Design review of the part built by this model. Coordinates are the model's own, in mm. Face numbers are marked on the shaded views. A direction names the side the tool comes from. Give positions to 0.01 mm unless a question says otherwise; leave off trailing zeros. Order: outer loops, then holes, each group sorted by start corner. A loop starts at its lowest first (then second) coordinate and runs counter-clockwise, first axis right, second up.
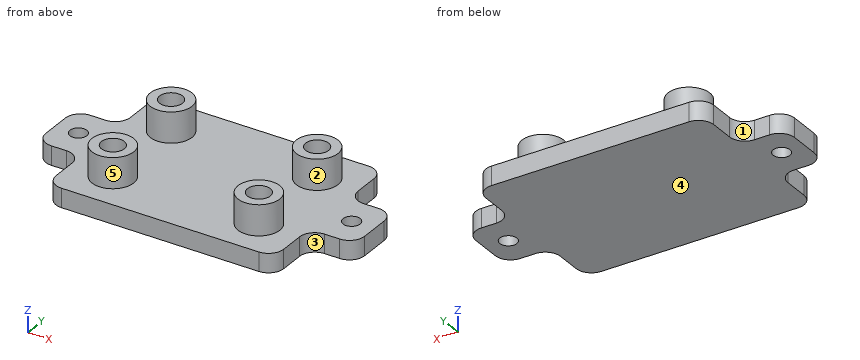
```python
from build123d import *

# Parameters (mm, degrees)
SKETCH1_W            = 60
SKETCH1_H            = 45
BOSS_EXTRUDE1_DEPTH  = 5
SKETCH3_R            = 5.5
SKETCH3_R_2          = 3.025
BOSS_EXTRUDE2_DEPTH  = 8
SKETCH4_W            = 12
SKETCH4_H            = 16
SKETCH4_R            = 2.55
BOSS_EXTRUDE3_DEPTH  = 5
FILLET1_R            = 4
M4_CLEARANCE_HOLE1_D = 4.5
MIRROR1_OUTLINE_R    = 2.25
MIRROR1_DEPTH        = 5
FILLET2_R            = 4


# Read off the part's stored shape, not the designer's step: Mirror1
with BuildPart() as part:
    # Sketch1 → Boss-Extrude1 (new body)
    with BuildSketch(Plane.XY):
        Rectangle(SKETCH1_W, SKETCH1_H)
    extrude(amount=BOSS_EXTRUDE1_DEPTH)

    # Sketch3 → Boss-Extrude2 (add)
    # profile 1 of 4: a face of its own
    with BuildSketch(Plane.XY.offset(5)):
        with Locations((-19.2405, 11.938)):
            Circle(SKETCH3_R)
        with Locations((-19.2405, 11.938)):
            Circle(SKETCH3_R_2, mode=Mode.SUBTRACT)
    # profile 2 of 4: a face of its own
    with BuildSketch(Plane.XY.offset(5)):
        with Locations((-19.2405, -11.938)):
            Circle(SKETCH3_R)
        with Locations((-19.2405, -11.938)):
            Circle(SKETCH3_R_2, mode=Mode.SUBTRACT)
    # profile 3 of 4: a face of its own
    with BuildSketch(Plane.XY.offset(5)):
        with Locations((19.2405, 11.938)):
            Circle(SKETCH3_R)
        with Locations((19.2405, 11.938)):
            Circle(SKETCH3_R_2, mode=Mode.SUBTRACT)
    # profile 4 of 4: a face of its own
    with BuildSketch(Plane.XY.offset(5)):
        with Locations((19.2405, -11.938)):
            Circle(SKETCH3_R)
        with Locations((19.2405, -11.938)):
            Circle(SKETCH3_R_2, mode=Mode.SUBTRACT)
    extrude(amount=BOSS_EXTRUDE2_DEPTH)

    # Sketch4 → Boss-Extrude3 (add)
    # profile 1 of 2: a face of its own
    with BuildSketch(Plane.XY.offset(5)):
        with Locations((-36, 0)):
            Rectangle(SKETCH4_W, SKETCH4_H)
        with Locations((-36, 0)):
            Circle(SKETCH4_R, mode=Mode.SUBTRACT)
    # profile 2 of 2: a face of its own
    with BuildSketch(Plane.XY.offset(5)):
        with Locations((-36, 0)):
            Circle(SKETCH4_R)
    extrude(amount=-BOSS_EXTRUDE3_DEPTH)

    # Fillet1
    fillet1_edges = [part.edges().sort_by_distance(p)[0] for p in [
        (-42, -8, 2.5),
        (-42, 8, 2.5),
        (-30, 8, 2.5),
        (-30, -8, 2.5),
        (-30, 22.5, 2.5),
        (-30, -22.5, 2.5),
    ]]
    fillet(fillet1_edges, radius=FILLET1_R)

    # M4 Clearance Hole1 (through all)
    with Locations(Plane.XY.offset(5)):
        with Locations((-36, 0)):
            Hole(M4_CLEARANCE_HOLE1_D / 2)

    # Mirror1 outline → Mirror1 (add)
    with BuildSketch(Plane.XY):
        with BuildLine():
            ThreePointArc((42, 4), (40.828427125, 6.828427125), (38, 8))
            Line((38, 8), (30, 8))
            Line((30, 8), (30, -8))
            Line((30, -8), (38, -8))
            ThreePointArc((38, -8), (40.828427125, -6.828427125), (42, -4))
            Line((42, -4), (42, 4))
        make_face()
        with Locations((36, 0)):
            Circle(MIRROR1_OUTLINE_R, mode=Mode.SUBTRACT)
    extrude(amount=MIRROR1_DEPTH)

    # Fillet2
    fillet2_edges = [part.edges().sort_by_distance(p)[0] for p in [
        (30, -8, 2.5),
        (30, 8, 2.5),
        (30, 22.5, 2.5),
        (30, -22.5, 2.5),
    ]]
    fillet(fillet2_edges, radius=FILLET2_R)


solid = part.part
```
1. For line 1 along Y through (x, z) = (36, 1.2); line 2 along X through (y, z) = (1, 2.25); line 3 along X through (y, z) = (-13.5, 1), list the stretches that pass through material, from the lowest coordinate up.
Recorded:
line 1: y = -8 to -2.25, 2.25 to 8
line 2: x = -42 to -38.02, -33.98 to 33.98, 38.02 to 42
line 3: x = -30 to 30
2. Take a section at C-C (z = 7.25). State how many separate pieces and enclosed holes the cut face has, then the cut area to 3 significant figures.
Recorded:
separate pieces: 4
enclosed holes: 4
area: 265 mm2
3. Take a section at D-D (y = -16). State the section outline as (x, z) points.
Recorded:
outline: (-30, 0) - (30, 0) - (30, 5) - (22.95, 5) - (22.95, 13) - (15.53, 13) - (15.53, 5) - (-15.53, 5) - (-15.53, 13) - (-22.95, 13) - (-22.95, 5) - (-30, 5) - close
4. Draft analysis for pull direction Y (two halves, no side actions). For the marked faces 3, 4 and 5, state which applies: pulls with the +Y half, pulls with the -Y half, needs draft (parallel to the pull), parting line crosses it, or undercut.
Recorded:
face 3: pulls with the -Y half
face 4: needs draft
face 5: undercut
5. Take a section at B-B (y = 0). State the section outline as (x, z) points, then the cut area to 3 significant figures.
Recorded:
outline: (-42, 0) - (-38.25, 0) - (-38.25, 5) - (-42, 5) - close; (-33.75, 0) - (33.75, 0) - (33.75, 5) - (-33.75, 5) - close; (38.25, 0) - (42, 0) - (42, 5) - (38.25, 5) - close
area: 375 mm2
6. For pin 1 (1.5 mm diameter, centred on y = -15, z = 1.5, fed in from +X); pin 2 (6.5 mm diameter, centred on x = -18, y = -11.5, fed in from +Z); pin 3 (4 mm diameter, centred on x = -36, y = 0, fed in from +Z); pin 4 (3 mm diameter, centred on x = -19.5, y = 11.5, fed in from +Z), all flat-tipped, find the tip position at first contact; note any pin that passes through.
Recorded:
pin 1: stops at x = 30
pin 2: stops at z = 13
pin 3: passes through
pin 4: stops at z = 5
7. Take a section at A-A (x = -36). State the section outline as (y, z) points, then the cut area to 3 significant figures.
Recorded:
outline: (-8, 0) - (-2.25, 0) - (-2.25, 5) - (-8, 5) - close; (2.25, 0) - (8, 0) - (8, 5) - (2.25, 5) - close
area: 57.5 mm2
8. Machinability: for the marked faces 1 and 2, which of the approach directions +Z, -Z, +X, -X, +Y, -Y give a long, thin tool a straight path to every point of the face, cutting with its end or side? Answer none if there is none.
Recorded:
face 1: +Z, -Z, -X, +Y
face 2: +Z
